```python
from build123d import *

# Parameters (mm, degrees)
EXTRUDE_1_DEPTH     = 100
SKETCH_3_R          = 3.2
CUT_EXTRUDE_1_DEPTH = 8
SKETCH_4_R          = 3.18
EXTRUDE_2_DEPTH     = 5.1


with BuildPart() as part:
    # 草图2 → 凸台-拉伸1 (new body)
    with BuildSketch(Plane(origin=(0, 0, 0), x_dir=(0, 0, -1), z_dir=(1, 0, 0))):
        with BuildLine():
            Line((-20.95, -1.45), (-8.95, -1.45))
            Line((-8.95, -1.45), (-8.95, -4.4))
            Line((-8.95, -4.4), (-29, -4.4))
            ThreePointArc((-29, -4.4), (-29.707106781, -4.692893219), (-30, -5.4))
            Line((-30, -5.4), (-30, -7.4))
            ThreePointArc((-30, -7.4), (-29.707106781, -8.107106781), (-29, -8.4))
            Line((-29, -8.4), (29, -8.4))
            ThreePointArc((29, -8.4), (29.707106781, -8.107106781), (30, -7.4))
            Line((30, -7.4), (30, -5.4))
            ThreePointArc((30, -5.4), (29.707106781, -4.692893219), (29, -4.4))
            Line((29, -4.4), (8.95, -4.4))
            Line((8.95, -4.4), (8.95, -1.45))
            Line((8.95, -1.45), (20.95, -1.45))
            ThreePointArc((20.95, -1.45), (21.657106781, -1.157106781), (21.95, -0.45))
            Line((21.95, -0.45), (21.95, 0.45))
            ThreePointArc((21.95, 0.45), (21.657106781, 1.157106781), (20.95, 1.45))
            Line((20.95, 1.45), (-20.95, 1.45))
            ThreePointArc((-20.95, 1.45), (-21.657106781, 1.157106781), (-21.95, 0.45))
            Line((-21.95, 0.45), (-21.95, -0.45))
            ThreePointArc((-21.95, -0.45), (-21.657106781, -1.157106781), (-20.95, -1.45))
        make_face()
    extrude(amount=EXTRUDE_1_DEPTH)

    # 草图3 → 切除-拉伸1 (cut)
    with BuildSketch(Plane(origin=(0, 1.45, 0), x_dir=(1, 0, 0), z_dir=(0, 1, 0))):
        with Locations(Location((11.492995831, 14, 0), (0, 0, 270))):
            Circle(SKETCH_3_R)
        with Locations(Location((24.492995831, 14, 0), (0, 0, 270))):
            Circle(SKETCH_3_R)
        with Locations(Location((37.492995831, 14, 0), (0, 0, 270))):
            Circle(SKETCH_3_R)
        with Locations(Location((50.492995831, 14, 0), (0, 0, 270))):
            Circle(SKETCH_3_R)
        with Locations(Location((63.492995831, 14, 0), (0, 0, 270))):
            Circle(SKETCH_3_R)
        with Locations(Location((76.492995831, 14, 0), (0, 0, 270))):
            Circle(SKETCH_3_R)
        with Locations(Location((89.492995831, 14, 0), (0, 0, 270))):
            Circle(SKETCH_3_R)
        with Locations(Location((89.492995831, -14, 0), (0, 0, 90))):
            Circle(SKETCH_3_R)
        with Locations(Location((76.492995831, -14, 0), (0, 0, 90))):
            Circle(SKETCH_3_R)
        with Locations(Location((63.492995831, -14, 0), (0, 0, 90))):
            Circle(SKETCH_3_R)
        with Locations(Location((50.492995831, -14, 0), (0, 0, 90))):
            Circle(SKETCH_3_R)
        with Locations(Location((37.492995831, -14, 0), (0, 0, 90))):
            Circle(SKETCH_3_R)
        with Locations(Location((24.492995831, -14, 0), (0, 0, 90))):
            Circle(SKETCH_3_R)
        with Locations(Location((11.492995831, -14, 0), (0, 0, 90))):
            Circle(SKETCH_3_R)
    extrude(amount=-CUT_EXTRUDE_1_DEPTH, mode=Mode.SUBTRACT)

    # 草图4 → 凸台-拉伸2 (add)
    with BuildSketch(Plane.XZ.offset(8.4)):
        with Locations(Location((11.9, 12.7, 0), (0, 0, 90))):
            Circle(SKETCH_4_R)
        with Locations(Location((37.3, 12.7, 0), (0, 0, 90))):
            Circle(SKETCH_4_R)
        with Locations(Location((62.7, 12.7, 0), (0, 0, 90))):
            Circle(SKETCH_4_R)
        with Locations(Location((88.1, 12.7, 0), (0, 0, 90))):
            Circle(SKETCH_4_R)
        with Locations(Location((62.7, -12.7, 0), (0, 0, 90))):
            Circle(SKETCH_4_R)
        with Locations(Location((37.3, -12.7, 0), (0, 0, 90))):
            Circle(SKETCH_4_R)
        with Locations(Location((11.9, -12.7, 0), (0, 0, 90))):
            Circle(SKETCH_4_R)
        with Locations(Location((88.1, -12.7, 0), (0, 0, 90))):
            Circle(SKETCH_4_R)
    extrude(amount=EXTRUDE_2_DEPTH)


solid = part.part
```
The model under review builds one solid part; all positions refer to its coordinate system, in mm. A direction names the side the tool comes from. Round coordinates to 2 decimals unless told otherwise and drop trailing zeros. Loops run counter-clockwise (first coordinate to the right, second up) from the corner with the lowest first, then second, coordinate; pieces in that order, holes last.
Item 1: Take a section at B-B (y = -10.25). Write out the cut boundary in (x, z), then the cut area to 3 significant figures.
Determined:
outline: circle Ø6.36 at (11.9, -12.7); circle Ø6.36 at (11.9, 12.7); circle Ø6.36 at (37.3, -12.7); circle Ø6.36 at (37.3, 12.7); circle Ø6.36 at (62.7, -12.7); circle Ø6.36 at (62.7, 12.7); circle Ø6.36 at (88.1, -12.7); circle Ø6.36 at (88.1, 12.7)
area: 254 mm2
Item 2: Take a section at A-A (z = 20). Write out the cut boundary in (x, y).
Determined:
outline: (0, -8.4) - (100, -8.4) - (100, -4.4) - (0, -4.4) - close; (0, -1.45) - (100, -1.45) - (100, 1.45) - (0, 1.45) - close
Item 3: Mouldability with a two-part tool opening along Z and no side actions: class faces 6 (the face through (49, -6, -30)), 7 (the face through (12, -13.5, 13)), 8 (the face through (66.33, 0.02, 12.52)), 9 (the face through (66.666, 0.02, -14.417)) as released by +Z, released by -Z, zero draft, split by the parting line, or undercut.
Determined:
face 6: released by -Z
face 7: zero draft
face 8: undercut
face 9: undercut
Item 4: For faces 1 (the face through (49, -6, 30)), 2 (the face through (12, -6.55, -14)), 3 (the face through (0, -3, 0)), 4 (the face through (84.947, -10.914, -13.114)), 5 (the face through (49, -4.4, -19)), list the 3-axis set-ups (+Z, -Z, +X, -X, +Y, -Y) from which the entire face can be reached by the end or side of a thin tool; tool diameter is ignored.
Determined:
face 1: +Z, +X, -X, +Y, -Y
face 2: +Y
face 3: +Z, -Z, -X, +Y, -Y
face 4: -Y
face 5: -Z, +X, -X
Item 5: For line 1 (Y direction, x = 73.5, z = -17.5); line 2 (Z direction, x = 30.5, y = -2.5); line 3 (Z direction, x = 18, y = -0.5), list the stretches that pass through material, from the lowest coordinate up.
Determined:
line 1: y = -8.4 to -4.4, -1.45 to 1.45
line 2: z = -8.95 to 8.95
line 3: z = -21.95 to 21.95
Item 6: Take a section at C-C (x = 18). Write out the cut boundary in (y, z), then the cut area to 3 significant figures.
Determined:
outline: (-8.4, -29) arc R1 ccw to (-7.4, -30) - (-5.4, -30) arc R1 ccw to (-4.4, -29) - (-4.4, -8.95) - (-1.45, -8.95) - (-1.45, -20.95) arc R1 ccw to (-0.45, -21.95) - (0.45, -21.95) arc R1 ccw to (1.45, -20.95) - (1.45, 20.95) arc R1 ccw to (0.45, 21.95) - (-0.45, 21.95) arc R1 ccw to (-1.45, 20.95) - (-1.45, 8.95) - (-4.4, 8.95) - (-4.4, 29) arc R1 ccw to (-5.4, 30) - (-7.4, 30) arc R1 ccw to (-8.4, 29) - close
area: 418 mm2
Item 7: Take a section at D-D (z = -8). Write out the cut boundary in (x, y).
Determined:
outline: (0, -8.4) - (100, -8.4) - (100, 1.45) - (0, 1.45) - close
Item 8: Clearance check with a flat-ended pin moving along its axis: pin 1 Ø5 at (x, z) = (50.49, -14) entering from +Y. State where the tip first meets the part, or that it passes through.
Determined:
pin 1: stops at y = -6.55
